Answer from the drawing. Dimensions are ordinates in mm from the lowest x, y and z of the part. Give positions to 0.01 mm unless a question says otherwise; leave off trailing zeros. Loops run counter-clockwise (first coordinate to the right, second up) from the corner with the lowest first, then second, coordinate; pieces in that order, holes last.
Item 1: The mould has two halves that part along X. Classify the marked faces 1, 2 and 3: pulls with the +X half, pulls with the -X half, needs draft (parallel to the pull), parting line crosses it, or undercut.
Item 2: Consider line 1 along Y through (x, z) = (25, 11.5); line 2 along Y through (x, z) = (21.5, 8.25); line 3 along X through (y, z) = (23.5, 19). Determine where each line is inside the solid, lowest interval first.
Item 3: Each of these flat-tipped pins is pushed along its axis until it touches: pin 1 Ø1 at (x, z) = (41.5, 4.5) entering from -Y; pin 2 Ø3 at (x, z) = (7, 19.5) entering from -Y; pin 3 Ø2 at (x, z) = (29, 9) entering from -Y. Where does it stop, or does it pass through?
Item 4: Section D-D, the plane x = 7 is taken. Give the vertices of the cut face in (y, z), and give its area (3 significant figures).
Item 5: Section A-A, the plane x = 25 is taken. Give the vertices of the cut face in (y, z), and give its area (3 significant figures).
Item 6: Section B-B, the plane y = 123 is taken. Give the vertices of the cut face in (x, z).
Item 7: Section C-C, the plane z = 22 is taken. Give the vertices of the cut face in (x, y).
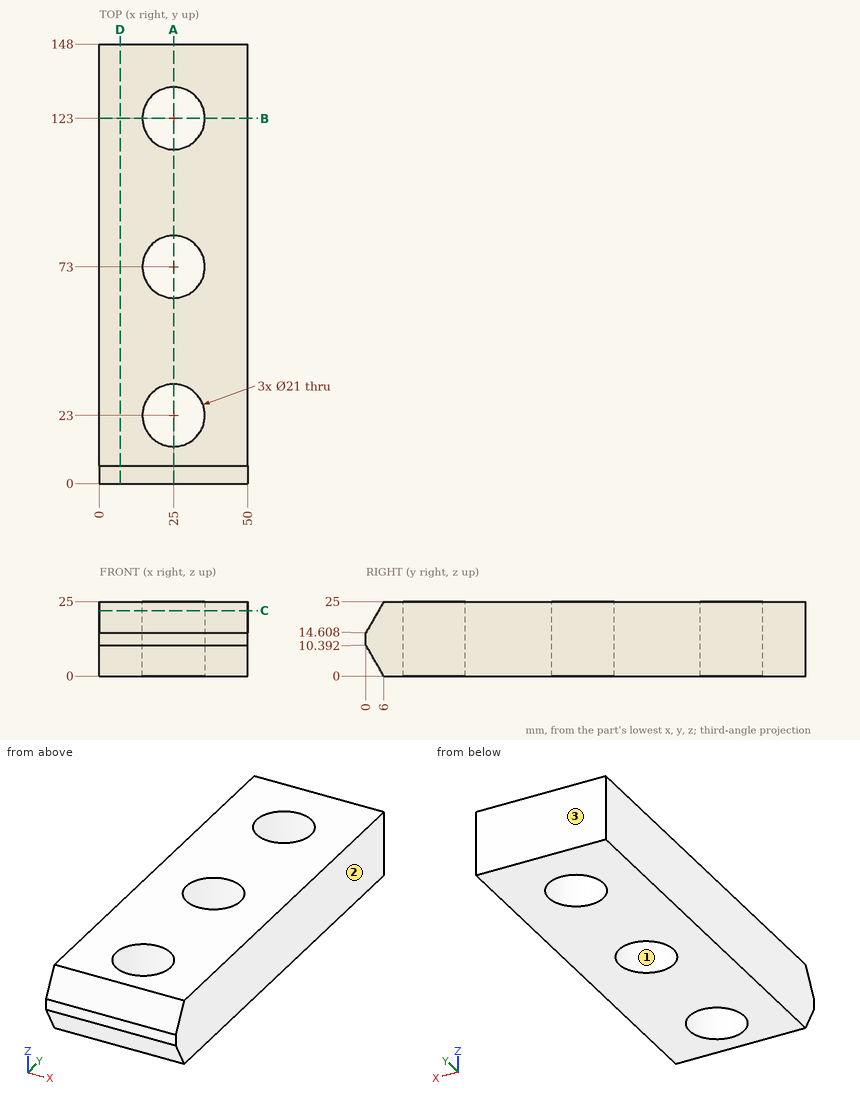
Worked answers:
1. face 1: undercut
1. face 2: pulls with the +X half
1. face 3: needs draft
2. line 1: y = 0 to 12.5, 33.5 to 62.5, 83.5 to 112.5, 133.5 to 148
2. line 2: y = 1.24 to 13.1, 32.9 to 63.1, 82.9 to 113.1, 132.9 to 148
2. line 3: x = 0 to 14.51, 35.49 to 50
3. pin 1: stops at y = 3.11
3. pin 2: stops at y = 1.96
3. pin 3: stops at y = 0.23
4. outline: (0, 10.39) - (6, 0) - (148, 0) - (148, 25) - (6, 25) - (0, 14.61) - close
4. area: 3,640 mm2
5. outline: (0, 10.39) - (6, 0) - (12.5, 0) - (12.5, 25) - (6, 25) - (0, 14.61) - close; (33.5, 0) - (62.5, 0) - (62.5, 25) - (33.5, 25) - close; (83.5, 0) - (112.5, 0) - (112.5, 25) - (83.5, 25) - close; (133.5, 0) - (148, 0) - (148, 25) - (133.5, 25) - close
5. area: 2,060 mm2
6. outline: (0, 0) - (14.5, 0) - (14.5, 25) - (0, 25) - close; (35.5, 0) - (50, 0) - (50, 25) - (35.5, 25) - close
7. outline: (0, 4.27) - (50, 4.27) - (50, 148) - (0, 148) - close; hole circle Ø21 at (25, 23); hole circle Ø21 at (25, 73); hole circle Ø21 at (25, 123)
